Build history of the part. All positions in model axes, mm. A direction names the side the tool comes from. Coordinates: 2 decimals unless noted, no trailing zeros. Write each loop counter-clockwise with the first axis right and the second up, starting at its lowest first coordinate (ties: lowest second). Pieces come first, ordered by that corner, then holes.
```python
from build123d import *

# Parameters (mm, degrees)
SKETCH_1_W          = 12
SKETCH_1_H          = 22.2
EXTRUDE_1_DEPTH     = 4
SKETCH_2_R          = 2.16
SKETCH_2_R_2        = 2.155
CUT_EXTRUDE_1_DEPTH = 4
CUT_EXTRUDE_2_DEPTH = 1.5
SKETCH_5_W          = 13.387393305
SKETCH_5_H          = 3.9
CUT_EXTRUDE_3_DEPTH = 14.23669143
SKETCH_6_W          = 12
SKETCH_6_H          = 7.85
EXTRUDE_3_DEPTH     = 4
SKETCH_7_W          = 12
SKETCH_7_H          = 4
EXTRUDE_4_DEPTH     = 20
SKETCH_8_R          = 1.5
CUT_EXTRUDE_4_DEPTH = 34.205760042


with BuildPart() as part:
    # 草图1 → 凸台-拉伸1 (new body)
    with BuildSketch(Plane.XY):
        Rectangle(SKETCH_1_W, SKETCH_1_H)
    extrude(amount=EXTRUDE_1_DEPTH)

    # 草图2 → 切除-拉伸1 (cut)
    with BuildSketch(Plane.XY.offset(4)):
        with Locations((1.7, -6.8)):
            Circle(SKETCH_2_R)
        with Locations((1.7, 2.9)):
            Circle(SKETCH_2_R_2)
    extrude(amount=-CUT_EXTRUDE_1_DEPTH, mode=Mode.SUBTRACT)

    # 草图4 → 切除-拉伸2 (cut)
    with BuildSketch(Plane(origin=(0, 0, 0), x_dir=(-1, 0, 0), z_dir=(0, 0, -1))):
        Polygon((-6, -1.4), (-6, -2.5), (-1.7, -2.5), (6, -2.5), (6, -1.4), (-1.7, -1.4), align=None)
    extrude(amount=-CUT_EXTRUDE_2_DEPTH, mode=Mode.SUBTRACT)

    # 草图5 → 切除-拉伸3 (cut, through all)
    with BuildSketch(Plane(origin=(0, 0, 0), x_dir=(-1, 0, 0), z_dir=(0, 0, -1))):
        with Locations((0.693696653, 9.15)):
            Rectangle(SKETCH_5_W, SKETCH_5_H)
    extrude(amount=-CUT_EXTRUDE_3_DEPTH, mode=Mode.SUBTRACT)

    # 草图6 → 凸台-拉伸3 (add)
    with BuildSketch(Plane.XY.offset(4)):
        with Locations((0, 11.125)):
            Rectangle(SKETCH_6_W, SKETCH_6_H)
    extrude(amount=-EXTRUDE_3_DEPTH)

    # 草图7 → 凸台-拉伸4 (add)
    with BuildSketch(Plane.XY.offset(4)):
        with Locations((0, 13.05)):
            Rectangle(SKETCH_7_W, SKETCH_7_H)
    extrude(amount=EXTRUDE_4_DEPTH)

    # 草图8 → 切除-拉伸4 (cut, through all)
    with BuildSketch(Plane.XZ.offset(-11.05)):
        with Locations(Location((0, 10, 0), (0, 0, 270))):
            Circle(SKETCH_8_R)
        with Locations(Location((0, 17, 0), (0, 0, 270))):
            Circle(SKETCH_8_R)
    extrude(amount=-CUT_EXTRUDE_4_DEPTH, mode=Mode.SUBTRACT)


solid = part.part
```
1. Saw through at D-D on y = -5.5. List the corners of the cut face in (x, z) (3 decimals).
Computed values:
outline: (-6, 0) - (-0.025, 0) - (-0.025, 4) - (-6, 4) - close; (3.425, 0) - (6, 0) - (6, 4) - (3.425, 4) - close
2. Probe line 1 along Y through (x, z) = (1.7, 0.9) (3 decimals); line 2 along Y through (x, z) = (1.7, 2.35) (3 decimals); line 3 along X through (y, z) = (13.75, 10). List the from-to ranges inside material, lowest first.
Computed values:
line 1: y = -11.1 to -8.96, -4.64 to -2.5, -1.4 to 0.745, 5.055 to 15.05
line 2: y = -11.1 to -8.96, -4.64 to 0.745, 5.055 to 15.05
line 3: x = -6 to -1.5, 1.5 to 6
3. Saw through at B-B on y = 13.25. List the corners of the cut face in (x, z).
Computed values:
outline: (-6, 0) - (6, 0) - (6, 24) - (-6, 24) - close; hole circle Ø3 at (0, 10); hole circle Ø3 at (0, 17)
4. 3-axis set-ups, long thin cutter, end or side, ignore diameter. For faces 5 (the face through (0, 11.05, 14)), 6 (the face through (0, -1.4, 1)), 7 (the face through (0, -11.1, 2)): which of +Z, -Z, +X, -X, +Y, -Y reach the whole face in a straight line?
Computed values:
face 5: +Z, +X, -X, -Y
face 6: -Z, +X, -X
face 7: +Z, -Z, +X, -X, -Y
5. Flat gauge pins, fed straight in: pin 1 (0.6 mm diameter, centred on x = 3, y = -2, fed in from -Z); pin 2 (6 mm diameter, centred on x = 4, y = -7.5, fed in from +Z); pin 3 (5 mm diameter, centred on x = -4.5, z = 12, fed in from -Y). Where does each tip first touch, or does it go through?
Computed values:
pin 1: stops at z = 1.5
pin 2: stops at z = 4
pin 3: stops at y = 11.05
6. Mould opens along Z. For faces 1 (the face through (0, 0, 4)), 2 (the face through (-6, 6, 3)), 3 (the face through (0.07, 13.02, 11.5)), 4 (the face through (0.07, 13.02, 18.5)) say: +Z half, -Z half, draft (parallel to the pull), parting line (faces both ways), or undercut.
Computed values:
face 1: +Z half
face 2: draft
face 3: undercut
face 4: undercut
7. Saw through at A-A on z = 10. List the corners of the cut face in (x, y), plus the area to 3 significant figures.
Computed values:
outline: (-6, 11.05) - (-1.5, 11.05) - (-1.5, 15.05) - (-6, 15.05) - close; (1.5, 11.05) - (6, 11.05) - (6, 15.05) - (1.5, 15.05) - close
area: 36.0 mm2
8. Saw through at C-C on x = 0.75. List the corners of the cut face in (y, z), plus the area to 3 significant figures.
Computed values:
outline: (-11.1, 0) - (-8.74, 0) - (-8.74, 4) - (-11.1, 4) - close; (-4.86, 0) - (-2.5, 0) - (-2.5, 1.5) - (-1.4, 1.5) - (-1.4, 0) - (0.97, 0) - (0.97, 4) - (-4.86, 4) - close; (4.83, 0) - (15.05, 0) - (15.05, 8.7) - (11.05, 8.7) - (11.05, 4) - (4.83, 4) - close; (11.05, 11.3) - (15.05, 11.3) - (15.05, 15.7) - (11.05, 15.7) - close; (11.05, 18.3) - (15.05, 18.3) - (15.05, 24) - (11.05, 24) - close
area: 131 mm2
